Verification items for this drawing (mm, ordinates from the low corner). A direction names the side the tool comes from. Round coordinates to 2 decimals unless told otherwise and drop trailing zeros. Write each loop counter-clockwise with the first axis right and the second up, starting at its lowest first coordinate (ties: lowest second). Pieces come first, ordered by that corner, then holes. Notation, with made-up numbers: (27.5, 18) -> (54.5, 18) arc R12 cw to (54.5, 26) -> close; hole circle Ø3 at (19, -15). An arc over 180 degrees is marked (long way). Use one line per item in the form item = value. Start each with the question number.
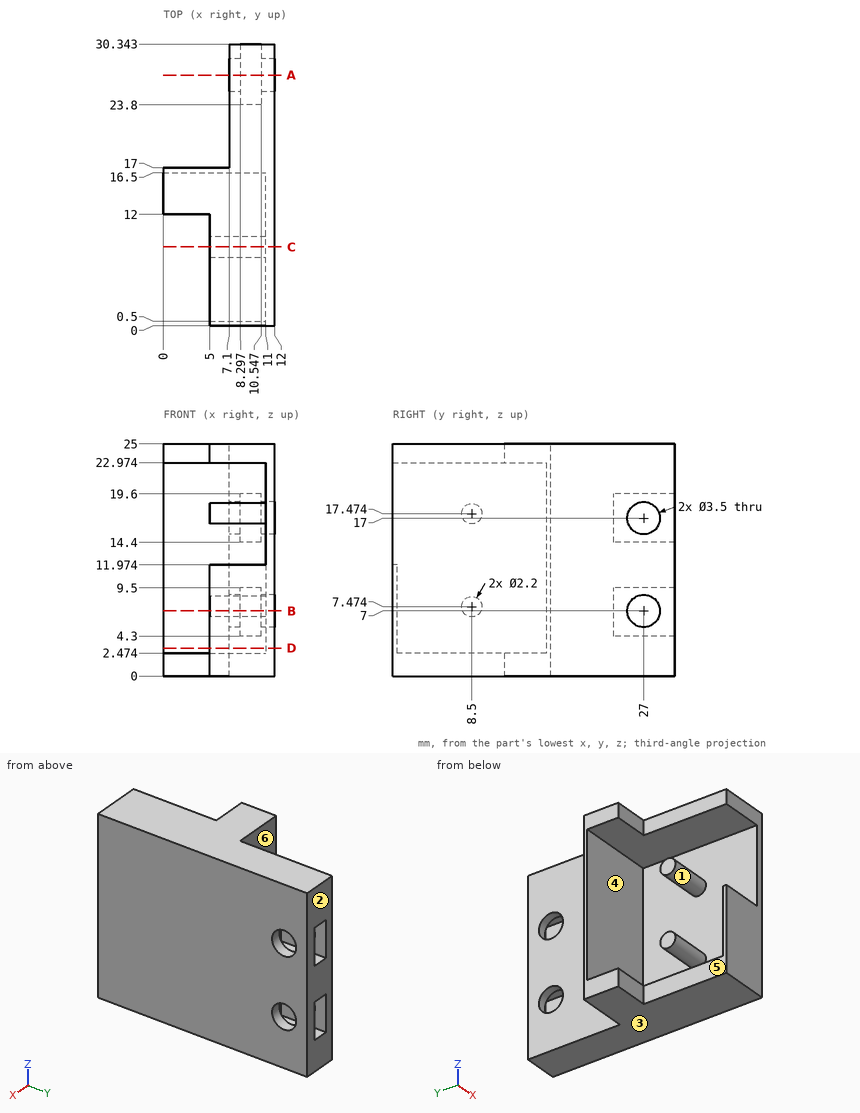
1. Scan lines: probe 1 along Z at (x, y) = (11.1, 27); probe 2 along Y at (x, z) = (5.5, 7.5); probe 3 along X at (y, z) = (8, 16.25). Record each from-to range of solid material in increasing order.
2. Sectioned sample at A-A (y = 27). Enter the section's corners in (x, z).
3. Sectioned sample at B-B (z = 7). Enter the section's corners in (x, y).
4. Sectioned sample at C-C (y = 8.5). Enter the section's corners in (x, z) (1 decimal).
5. Tool access check on the marked faces 4, 5 and 6. Record the directions out of +Z, -Z, +X, -X, +Y, -Y that give a thin tool (end or side, any length) a straight path to the whole face; none if there is none.
6. Depth check by flat-ended pin: pin 1 (0.7 mm diameter, centred on x = 9, z = 16.5, fed in from +Y); pin 2 (5 mm diameter, centred on y = 4, z = 8.5, fed in from -X); pin 3 (1.8 mm diameter, centred on y = 8.5, z = 7, fed in from -X). Enter the tip coordinate at first touch or a pass-through.
7. Sectioned sample at D-D (z = 3). Enter the section's corners in (x, y).
8. Mould release check, pull along Z, two halves, no side actions. Record for the marked faces 1, 2 and 3: +Z half, -Z half, draft (parallel to the pull), parting line (faces both ways), or undercut.
Returned:
q1.probe_1 = 0 to 5.25, 8.75 to 15.25, 18.75 to 25
q1.probe_2 = 0 to 0.5, 7.4 to 9.6, 16.5 to 17
q1.probe_3 = 11 to 12
q2.outline = (7.1, 0) -> (12, 0) -> (12, 5.25) -> (10.55, 5.25) -> (10.55, 4.3) -> (8.3, 4.3) -> (8.3, 5.25) -> (7.1, 5.25) -> close; (7.1, 8.75) -> (8.3, 8.75) -> (8.3, 9.5) -> (10.55, 9.5) -> (10.55, 8.75) -> (12, 8.75) -> (12, 15.25) -> (10.55, 15.25) -> (10.55, 14.4) -> (8.3, 14.4) -> (8.3, 15.25) -> (7.1, 15.25) -> close; (7.1, 18.75) -> (8.3, 18.75) -> (8.3, 19.6) -> (10.55, 19.6) -> (10.55, 18.75) -> (12, 18.75) -> (12, 25) -> (7.1, 25) -> close
q3.outline = (0, 16.5) -> (11, 16.5) -> (11, 9.49) -> (5, 9.49) -> (5, 7.51) -> (11, 7.51) -> (11, 0.5) -> (5, 0.5) -> (5, 0) -> (12, 0) -> (12, 25.25) -> (10.55, 25.25) -> (10.55, 23.8) -> (8.3, 23.8) -> (8.3, 25.25) -> (7.1, 25.25) -> (7.1, 17) -> (0, 17) -> close; (7.1, 28.75) -> (8.3, 28.75) -> (8.3, 30.34) -> (7.1, 30.34) -> close; (10.55, 28.75) -> (12, 28.75) -> (12, 30.34) -> (10.55, 30.34) -> close
q4.outline = (5, 0) -> (12, 0) -> (12, 25) -> (5, 25) -> (5, 23) -> (11, 23) -> (11, 18.6) -> (5, 18.6) -> (5, 16.4) -> (11, 16.4) -> (11, 8.6) -> (5, 8.6) -> (5, 6.4) -> (11, 6.4) -> (11, 2.5) -> (5, 2.5) -> close
q5.face_4 = -X
q5.face_5 = +Z, -Z, -X, -Y
q5.face_6 = +Z, -Z, -X, +Y
q6.pin_1 = 23.8
q6.pin_2 = 11
q6.pin_3 = 5
q7.outline = (0, 16.5) -> (11, 16.5) -> (11, 0.5) -> (5, 0.5) -> (5, 0) -> (12, 0) -> (12, 30.34) -> (7.1, 30.34) -> (7.1, 17) -> (0, 17) -> close
q8.face_1 = undercut
q8.face_2 = draft
q8.face_3 = -Z half
